Input: part model. Units: mm. Frame: model coordinates. A direction names the side the tool comes from. Give positions to 0.01 mm unless a question says otherwise; leave off trailing zeros. Loops run counter-clockwise (first coordinate to the right, second up) from the corner with the lowest first, then second, coordinate; pieces in that order, holes last. Notation, with made-up numbers: M 87,30 L 131,30 A30 ccw 131,53 Z; hole C 66.5,-33.5 d1. An arc over 180 degrees is marked long. Return JSON: item names as keys, results as strings. Group by question number.
```python
from build123d import *

# Parameters (mm, degrees)
SKETCH1_R           = 133.35
SKETCH1_R_2         = 110.49
BOSS_EXTRUDE1_DEPTH = 20.32
FILLET1_R           = 5.08
FILLET4_R           = 5.08
FILLET5_R           = 5.08
FILLET6_R           = 5.08
SKETCH2_R           = 25.4
BOSS_EXTRUDE2_DEPTH = 12.7
SKETCH3_R           = 11.43
BOSS_EXTRUDE3_DEPTH = 381
BOSS_EXTRUDE4_DEPTH = 25.4
SKETCH5_R           = 19.05
BOSS_EXTRUDE5_DEPTH = 12.7


with BuildPart() as part:
    # Sketch1 → Boss-Extrude1 (new body)
    with BuildSketch(Plane.XY):
        Circle(SKETCH1_R)
        Circle(SKETCH1_R_2, mode=Mode.SUBTRACT)
    extrude(amount=BOSS_EXTRUDE1_DEPTH)

    # Fillet1
    fillet1_edges = [part.edges().sort_by_distance(p)[0] for p in [
        (-133.35, 0, 20.32),
    ]]
    fillet(fillet1_edges, radius=FILLET1_R)

    # Fillet4
    fillet4_edges = [part.edges().sort_by_distance(p)[0] for p in [
        (-133.35, 0, 0),
    ]]
    fillet(fillet4_edges, radius=FILLET4_R)

    # Fillet5
    fillet5_edges = [part.edges().sort_by_distance(p)[0] for p in [
        (-110.49, 0, 20.32),
    ]]
    fillet(fillet5_edges, radius=FILLET5_R)

    # Fillet6
    fillet6_edges = [part.edges().sort_by_distance(p)[0] for p in [
        (-110.49, 0, 0),
    ]]
    fillet(fillet6_edges, radius=FILLET6_R)



with BuildPart() as body_2:
    # Sketch2 → Boss-Extrude2 (new body)
    with BuildSketch(Plane.XY.offset(20.32)):
        with BuildLine():
            add(Edge.make_bspline(
                [(111.995773379, 28.519671196), (108.395461325, 33.640925655), (103.465758881, 38.766955506)],
                knots=[0.86323948, 0.86323948, 0.86323948, 1, 1, 1], degree=2))
            Line((103.465758881, 38.766955506), (17.465361403, 18.442373791))
            ThreePointArc((17.465361403, 18.442373791), (23.332168562, 10.038421698), (25.4, 0))
            ThreePointArc((25.4, 0), (23.332168562, -10.038421698), (17.465361403, -18.442373791))
            Line((17.465361403, -18.442373791), (104.480917214, -35.941313806))
            add(Edge.make_bspline(
                [(104.480917214, -35.941313806), (109.199570697, -30.926942984), (112.628608991, -25.907939648)],
                knots=[0, 0, 0, 0.134699054, 0.134699054, 0.134699054], degree=2))
            ThreePointArc((112.628608991, -25.907939648), (114.832297811, -13.037188327), (115.57, 0))
            ThreePointArc((115.57, 0), (114.672962004, 14.37138425), (111.995773379, 28.519671196))
        make_face()
        with BuildLine():
            ThreePointArc((-17.465361403, 18.442373791), (0, 25.4), (17.465361403, 18.442373791))
            Line((17.465361403, 18.442373791), (41.120888712, 102.55297466))
            add(Edge.make_bspline(
                [(33.408134269, 110.6359863), (37.257292789, 107.035833442), (41.120888712, 102.55297466)],
                knots=[0.898413925, 0.898413925, 0.898413925, 1, 1, 1], degree=2))
            ThreePointArc((33.408134269, 110.6359863), (3.618968694, 115.513323758), (-26.417084957, 112.510277408))
            add(Edge.make_bspline(
                [(-33.5455644, 105.274570572), (-29.987921782, 109.295772293), (-26.417084957, 112.510277408)],
                knots=[0, 0, 0, 0.097113874, 0.097113874, 0.097113874], degree=2))
            Line((-33.5455644, 105.274570572), (-17.465361403, 18.442373791))
        make_face()
        with BuildLine():
            Line((41.120888883, -102.552974591), (17.465361403, -18.442373791))
            ThreePointArc((17.465361403, -18.442373791), (0, -25.4), (-17.465361403, -18.442373791))
            Line((-17.465361403, -18.442373791), (-33.545564575, -105.274570516))
            add(Edge.make_bspline(
                [(-33.545564575, -105.274570516), (-26.738144431, -110.571915765), (-19.922448027, -113.839891798)],
                knots=[0, 0, 0, 0.182948004, 0.182948004, 0.182948004], degree=2))
            ThreePointArc((-19.922448027, -113.839891798), (3.568860133, -115.514882753), (26.911965601, -112.392931306))
            add(Edge.make_bspline(
                [(26.911965601, -112.392931306), (34.011973832, -108.564945177), (41.120888883, -102.552974591)],
                knots=[0.810210618, 0.810210618, 0.810210618, 1, 1, 1], degree=2))
        make_face()
        with BuildLine():
            ThreePointArc((-17.465361403, -18.442373791), (-25.4, 0), (-17.465361403, 18.442373791))
            Line((-17.465361403, 18.442373791), (-103.453712161, 38.799092001))
            add(Edge.make_bspline(
                [(-111.872978372, 28.997613871), (-108.286344087, 33.895850119), (-103.453712161, 38.799092001)],
                knots=[0.869248391, 0.869248391, 0.869248391, 1, 1, 1], degree=2))
            ThreePointArc((-111.872978372, 28.997613871), (-115.56181287, 1.375611191), (-112.531537583, -26.326373643))
            add(Edge.make_bspline(
                [(-104.492035357, -35.908977246), (-109.115451856, -31.120100592), (-112.531537583, -26.326373643)],
                knots=[0, 0, 0, 0.128706822, 0.128706822, 0.128706822], degree=2))
            Line((-104.492035357, -35.908977246), (-17.465361403, -18.442373791))
        make_face()
        Circle(SKETCH2_R)
    extrude(amount=-BOSS_EXTRUDE2_DEPTH)


with BuildPart() as part_1:
    add(part.part)

    add(body_2.part)  # Boss-Extrude3 merges body 2
    # Sketch3 → Boss-Extrude3 (add)
    with BuildSketch(Plane.XY.offset(20.32)):
        Circle(SKETCH3_R)
    extrude(amount=BOSS_EXTRUDE3_DEPTH)

    # Sketch4 → Boss-Extrude4 (add)
    with BuildSketch(Plane.XY.offset(401.32)):
        with BuildLine():
            Line((0.984973427, -8.925344441), (0.984973427, -7.883058907))
            Line((0.984973427, -7.883058907), (-1.301026573, -7.883058907))
            Line((-1.301026573, -7.883058907), (-1.301026573, -8.884777763))
            ThreePointArc((-1.301026573, -8.884777763), (-6.277222362, -6.420936494), (-8.853056418, -1.501778309))
            Line((-8.853056418, -1.501778309), (-8.038471669, -1.501778309))
            Line((-8.038471669, -1.501778309), (-8.038471669, 0.784221691))
            Line((-8.038471669, 0.784221691), (-8.945218968, 0.784221691))
            ThreePointArc((-8.945218968, 0.784221691), (-6.582089434, 6.108031166), (-1.449428448, 8.861777655))
            Line((-1.449428448, 8.861777655), (-1.449428448, 7.87722015))
            Line((-1.449428448, 7.87722015), (0.836571552, 7.87722015))
            Line((0.836571552, 7.87722015), (0.836571552, 8.940475048))
            ThreePointArc((0.836571552, 8.940475048), (6.346995913, 6.351975198), (8.939816257, 0.84358244))
            Line((8.939816257, 0.84358244), (8.107652261, 0.84358244))
            Line((8.107652261, 0.84358244), (8.107652261, -1.44241756))
            Line((8.107652261, -1.44241756), (8.862921506, -1.44241756))
            ThreePointArc((8.862921506, -1.44241756), (6.18415777, -6.510617383), (0.984973427, -8.925344441))
        make_face()
    extrude(amount=BOSS_EXTRUDE4_DEPTH)

    # Sketch5 → Boss-Extrude5 (add)
    with BuildSketch(Plane.XY.offset(20.32)):
        Circle(SKETCH5_R)
    extrude(amount=BOSS_EXTRUDE5_DEPTH)


solid = part_1.part
```
Item 1: First-contact query: pin 1 Ø0.8 at (x, z) = (8.5, 410.5) entering from +Y; pin 2 Ø0.8 at (y, z) = (-8.5, 420) entering from +X; pin 3 Ø10 at (x, y) = (16.5, 102) entering from -Z. Flat tips, straight axial feed; report the tip coordinate or a pass-through.
Item 2: Section A-A, the plane z = 389.5. Return loops of the section in (x, y), then the cut area to 3 significant figures.
Item 3: Reachability of faces 1 (the face through (10.902, 3.433, 214.592)), 2 (the face through (-2, 2, 7.62)), 3 (the face through (-115, 20, 0)), 4 (the face through (29.128, 59.909, 14.059)) from +Z, -Z, +X, -X, +Y, -Y: full face, straight path, thin tool, end or side. Return the list, or none.
Item 4: Material intervals for line 1 (Y direction, x = 0, z = 7.5); line 2 (Z direction, x = -6.5, y = 77.5); line 3 (Y direction, x = 0, z = 11), sorted ascending. Write a range as from..to.
Item 5: Section B-B, the plane x = -64. Give the number of separate pieces and of enclosed holes in the cut face, then the cut area to 3 significant figures.
Item 6: Pull-direction query (Y, two-part tool) for faces 5 (the face through (-2, -27, 20.32)), 6 (the face through (50.984, -98.024, 8.96)), 7 (the face through (-15.12, -11.59, 26.58)); classes: pulls with the +Y half, pulls with the -Y half, needs draft (parallel to the pull), parting line crosses it, or undercut.
Answer below:
{
 "1": {"pin 1": "y = 3.88", "pin 2": "x = 3.88", "pin 3": "z = 7.62"},
 "2": {"outline": "C 0,0 d22.86", "area": "410 mm^2"},
 "3": {"face 1": "+Z", "face 2": "-Z", "face 3": "-Z, +X, -X, +Y, -Y", "face 4": "+Z, -Z"},
 "4": {"line 1": "-133.35..-110.49, 110.49..133.35", "line 2": "7.62..20.32", "line 3": "-133.35..133.35"},
 "5": {"separate pieces": "3", "enclosed holes": "0", "area": "1,770 mm^2"},
 "6": {"face 5": "needs draft", "face 6": "undercut", "face 7": "parting line crosses it"}
}
